Autodesk Inventor part; units mm, degrees
ref_plane "YZ Plane" through (0, 0, 0) normal (1, 0, 0) x (0, 1, 0)
ref_plane "XZ Plane" through (0, 0, 0) normal (0, 1, 0) x (-1, 0, 0)
ref_plane "XY Plane" through (0, 0, 0) normal (0, 0, 1) x (1, 0, 0)
sketch "Sketch1" plane through (0, 0, 0) normal (0, 0, 1) x (1, 0, 0)
  line L0 (0, 0) -> (44, 0)
  line L1 (44, 0) -> (44, 44)
  line L2 (44, 44) -> (0, 44)
  line L3 (0, 44) -> (0, 0)
  dimension "d0" = 44
  dimension "d1" = 44
extrude "Extrusion1" add sketch "Sketch1" along normal blind 4
chamfer "Chamfer1" distance 4 angle 45 4 edges at (22, 44, 4) (44, 22, 4) (22, 0, 4) (0, 22, 4)
sketch "Sketch2" plane through (0, 0, 4) normal (0, 0, 1) x (1, 0, 0)
  line L0 (40, 4) -> (4, 4)
  line L1 (40, 40) -> (40, 4)
  line L2 (4, 40) -> (40, 40)
  line L3 (4, 4) -> (4, 40)
  point P0 (0, 0)
extrude "Extrusion2" cut sketch "Sketch2" against normal blind 3.6
properties part number "clear-square-hollow"
Verification items for the finished model (mm, model axes). A direction names the side the tool comes from. Round coordinates to 2 decimals unless told otherwise and drop trailing zeros. Loops run counter-clockwise (first coordinate to the right, second up) from the corner with the lowest first, then second, coordinate; pieces in that order, holes last. Notation, with made-up numbers: (17.5, 28.25) - (74.5, 28.25) arc R15 cw to (74.5, 51.25) - close; hole circle Ø7 at (72, 38.25). An arc over 180 degrees is marked (long way). Use a Markdown table: item, result. Add a question column.
1. Section check A-A, the plane z = 3.15. Record the boundary of the cut face in (x, y), plus the area to 3 significant figures.
2. Thickness scan on probe 1 along Z at (x, y) = (21.5, 23); probe 2 along Y at (x, z) = (34.5, 0.85); probe 3 along X at (y, z) = (32.5, 1.75). Record the ranges inside material, lowest first. Write a range as [from, to].
3. Access from +Z, -Z, +X, -X, +Y, -Y to the whole of each face (thin tool, end or side, straight path). Record for faces 1 (the face through (4, 22, 2)), 2 (the face through (42, 22, 2)).
4. Release check for a two-part mould opening along X. For faces 3 (the face through (22, 40, 2)), 4 (the face through (2, 22, 2)), 5 (the face through (22, 42, 2)) record: released by +X, released by -X, zero draft, split by the parting line, or undercut.
5. Gauge pin test, flat ends, axial feed: pin 1 (1.5 mm diameter, centred on x = 24.5, z = 1, fed in from +Y); pin 2 (3 mm diameter, centred on x = 37, y = 7.5, fed in from +Z); pin 3 (2 mm diameter, centred on y = 8.5, z = 0.5, fed in from -X). Record the tip position at first contact, or that the pin passes through.
Checks:
| question | item | result |
|---|---|---|
| 1 | outline | (3.15, 3.15) - (40.85, 3.15) - (40.85, 40.85) - (3.15, 40.85) - close; hole (4, 4) - (40, 4) - (40, 40) - (4, 40) - close |
| 1 | area | 125 mm^2 |
| 2 | probe 1 | z = [0, 0.4] |
| 2 | probe 2 | y = [0.85, 4], [40, 43.15] |
| 2 | probe 3 | x = [1.75, 4], [40, 42.25] |
| 3 | face 1 | +Z |
| 3 | face 2 | +Z, +X, +Y, -Y |
| 4 | face 3 | undercut |
| 4 | face 4 | released by -X |
| 4 | face 5 | zero draft |
| 5 | pin 1 | stops at y = 43.75 |
| 5 | pin 2 | stops at z = 0.4 |
| 5 | pin 3 | stops at x = 0 |
